from build123d import *

# Parameters (mm, degrees)
SKETCH1_W           = 457.2
SKETCH1_H           = 457.2
BOSS_EXTRUDE1_DEPTH = 2.8321
SKETCH2_R           = 3.175
SKETCH2_R_2         = 19.05
SKETCH2_W           = 31.75
SKETCH2_H           = 31.75
CUT_EXTRUDE1_DEPTH  = 536.658532911


with BuildPart() as part:
    # Sketch1 → Boss-Extrude1 (new body)
    with BuildSketch(Plane.XY):
        with Locations((-50.8, -228.4095)):
            Rectangle(SKETCH1_W, SKETCH1_H)
    extrude(amount=BOSS_EXTRUDE1_DEPTH)

    # Sketch2 → Cut-Extrude1 (cut, through all)
    with BuildSketch(Plane.XY.offset(2.8321)):
        with Locations((-260.35, -18.8595)):
            Circle(SKETCH2_R)
        with Locations((-260.35, -437.9595)):
            Circle(SKETCH2_R)
        with Locations((158.75, -437.9595)):
            Circle(SKETCH2_R)
        with Locations((158.75, -18.8595)):
            Circle(SKETCH2_R)
        with Locations((19.00555, -387.1595)):
            Circle(SKETCH2_R_2)
        with Locations((-248.158, -113.6015)):
            Rectangle(SKETCH2_W, SKETCH2_H)
    extrude(amount=-CUT_EXTRUDE1_DEPTH, mode=Mode.SUBTRACT)


solid = part.part
Design review of the part built by this model. Coordinates are the model's own, in mm. Round coordinates to 2 decimals unless told otherwise and drop trailing zeros. One line per item, written item: value. Start each with the question number.
1) Draft analysis for pull direction X (two halves, no side actions). For faces 1 (the cylindrical face through (14.876, -405.756, 1.436)), 2 (the flat face through (-54, -225, 0)), state which applies: +X half, -X half, draft (parallel to the pull), parting line (faces both ways), or undercut.
2) Insertion check: pin 1 Ø4 at (x, y) = (158.75, -18.86) entering from +Z. The pin has a flat end and moves straight along its axis. Give the tip position at first contact, or say it passes through.
3) To check wall thickness, follow L1, parallel to Y at x = -260.35, z = 0.7; L2, parallel to Y at x = -254, z = 2.6; L3, parallel to X at y = -376.5, z = 1.9. State the ranges of each line that lie inside material, in increasing order. Write a range as from..to.
Reported:
1. face 1: undercut
1. face 2: draft
2. pin 1: passes through
3. L1: y = -457.01..-441.13, -434.78..-129.48, -97.73..-22.03, -15.68..0.19
3. L2: y = -457.01..-129.48, -97.73..0.19
3. L3: x = -279.4..3.22, 34.79..177.8
